The model under review builds one solid part; all positions refer to its coordinate system, in mm. A direction names the side the tool comes from. Give positions to 0.01 mm unless a question says otherwise; leave off trailing zeros. Write each loop counter-clockwise with the first axis right and the second up, starting at its lowest first coordinate (ties: lowest second). Pieces come first, ordered by that corner, then holes. Notation, with made-up numbers: M -38.5,-13.75 L -16.5,-13.75 A17 cw -16.5,-7.75 Z; hole C -11.75,19.5 d10. An arc over 180 degrees is marked long. Write item = value, one per line. Start each with the question number.
```python
from build123d import *

# Parameters (mm, degrees)
EXTRUDE_1_DEPTH     = 4.6
EXTRUDE_2_DEPTH     = 4.1
CUT_EXTRUDE_1_DEPTH = 26.767033201


with BuildPart() as part:
    # Эскиз1 → Бобышка-Вытянуть1 (new body)
    with BuildSketch(Plane.XY):
        with BuildLine():
            Line((0, 2.9), (15, 2.9))
            Line((15, 2.9), (15, -2.9))
            Line((15, -2.9), (0, -2.9))
            ThreePointArc((0, -2.9), (-2.9, 0), (0, 2.9))
        make_face()
    extrude(amount=EXTRUDE_1_DEPTH)

    # Эскиз2 → Бобышка-Вытянуть2 (add)
    with BuildSketch(Plane.XY.offset(4.6)):
        with BuildLine():
            Line((24, 3.5), (24, -3.5))
            Line((24, -3.5), (15, -3.5))
            Line((15, -3.5), (15, -2.9))
            Line((15, -2.9), (0, -2.9))
            ThreePointArc((0, -2.9), (-2.9, 0), (0, 2.9))
            Line((0, 2.9), (15, 2.9))
            Line((15, 2.9), (15, 3.5))
            Line((15, 3.5), (24, 3.5))
        make_face()
    extrude(amount=EXTRUDE_2_DEPTH)

    # Эскиз3 → Вырез-Вытянуть1 (cut, through all)
    with BuildSketch(Plane.XY.offset(8.7)):
        with BuildLine():
            Line((0, 1.6), (12.2, 1.6))
            ThreePointArc((12.2, 1.6), (13.8, 0), (12.2, -1.6))
            Line((12.2, -1.6), (0, -1.6))
            ThreePointArc((0, -1.6), (-1.6, 0), (0, 1.6))
        make_face()
    extrude(amount=-CUT_EXTRUDE_1_DEPTH, mode=Mode.SUBTRACT)


solid = part.part
```
Item 1: To check wall thickness, follow probe 1 along Y at (x, z) = (1.25, 1.25); probe 2 along X at (y, z) = (0, 4.25); probe 3 along Z at (x, y) = (23, -1.75). State the ranges of each line that lie inside material, in increasing order. Write a range as [from, to].
Item 2: The part is to be moulded in two halves that separate along X. For faces 6 (the flat face through (7, 2.9, 4)), 7 (the cylindrical face through (-2.9, -0.1, 4.3)), 8 (the flat face through (6, 1.6, 4)), 9 (the flat face through (15, 0, 2)), say which applies: released by +X, released by -X, zero draft, split by the parting line, or undercut.
Item 3: We need section A-A, the plane x = 5.75. Write out the cut boundary in (y, z).
Item 4: Clearance check with flat-ended pins moving along their axes: P1, Ø2, axis at x = 21, y = 2, coming from the -Z side; P2, Ø3.5, axis at y = 0.5, z = 2.5, coming from the +X side; P3, Ø0.7, axis at y = -3, z = 7, coming from the -X side. State where each tip first meets the part, or that it passes through.
Item 5: We need section B-B, the plane y = 0. Write out the cut boundary in (x, z), and give its area (4 significant figures).
Item 6: We need section C-C, the plane z = 2.5. Write out the cut boundary in (x, y), and give its area (3 significant figures).
Item 7: For faces 1 (the flat face through (8, -2.9, 4)), 2 (the flat face through (14, 1, 8.7)), 3 (the flat face through (19, 3.5, 7)), 4 (the cylindrical face through (13.8, 0, 4.4)), 5 (the flat face through (20, 0, 4.6)), list the 3-axis set-ups (+Z, -Z, +X, -X, +Y, -Y) from which the entire face can be reached by the end or side of a thin tool; tool diameter is ignored.
Item 8: We need section D-D, the plane x = 13.25. Write out the cut boundary in (y, z).
Worked out:
q1.probe_1 = [-2.9, -1.6], [1.6, 2.9]
q1.probe_2 = [-2.9, -1.6], [13.8, 15]
q1.probe_3 = [4.6, 8.7]
q2.face_6 = zero draft
q2.face_7 = released by -X
q2.face_8 = undercut
q2.face_9 = released by +X
q3.outline = M -2.9,0 L -1.6,0 L -1.6,8.7 L -2.9,8.7 Z; M 1.6,0 L 2.9,0 L 2.9,8.7 L 1.6,8.7 Z
q4.P1 = 4.6
q4.P2 = 15
q4.P3 = -1.18
q5.outline = M -2.9,0 L -1.6,0 L -1.6,8.7 L -2.9,8.7 Z; M 13.8,0 L 15,0 L 15,4.6 L 24,4.6 L 24,8.7 L 13.8,8.7 Z
q5.area = 58.65 mm²
q6.outline = M 0,-2.9 L 15,-2.9 L 15,2.9 L 0,2.9 A2.9 ccw Z; hole M 0,-1.6 L 12.2,-1.6 A1.6 ccw 12.2,1.6 L 0,1.6 A1.6 ccw Z
q6.area = 53.1 mm²
q7.face_1 = +Z, -Z, -X, -Y
q7.face_2 = +Z, +X, -X, +Y, -Y
q7.face_3 = +Z, -Z, +X, -X, +Y
q7.face_4 = +Z, -Z
q7.face_5 = -Z, +X, +Y, -Y
q8.outline = M -2.9,0 L -1.21,0 L -1.21,8.7 L -2.9,8.7 Z; M 1.21,0 L 2.9,0 L 2.9,8.7 L 1.21,8.7 Z
